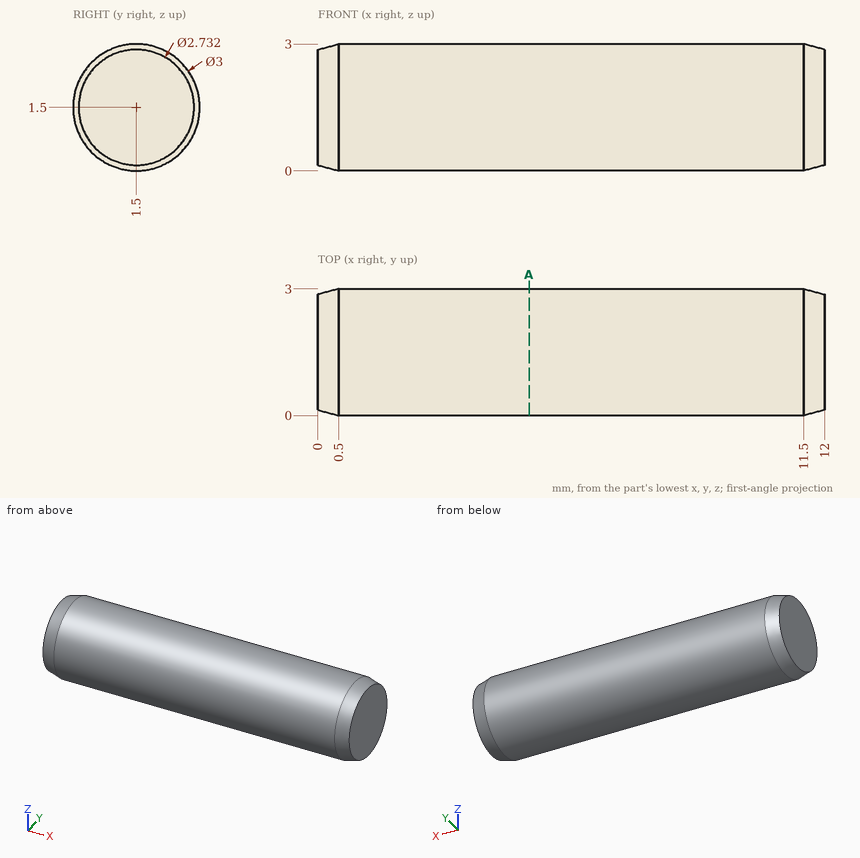
Geometry: see drawing. Coordinates: mm, zero at the bounding-box minimum. Coordinates: 2 decimals unless noted, no trailing zeros. Order: outer loops, then holes, each group sorted by start corner. A loop starts at its lowest first (then second) coordinate and runs counter-clockwise, first axis right, second up. Notation, with made-up numbers: M 7.5,23.5 L 19.5,23.5 A19 ccw 19.5,58.5 Z; hole C -5,64.25 d10. An arc over 180 degrees is marked long. Write each question's results on one line, items separated by ' | '. Start each with the question number.
1) Line query: line 1 (Z direction, x = 2.5, y = 1.4); line 2 (Z direction, x = 2.75, y = 2.65). Output: solid intervals per line, ascending. Write a range as from..to.
2) Contact query for a flat-ended pin moving along its axis: pin 1 Ø1.5 at (x, y) = (10.5, 1) entering from +Z. Output: stop coordinate, or through.
3) Section query A-A (x = 5). Return the cut outline in (y, z), plus the area to 3 significant figures.
Answers:
1) line 1: z = 0..3 | line 2: z = 0.54..2.46
2) pin 1: stops at z = 3
3) outline: C 1.5,1.5 d3 | area: 7.07 mm^2
